CAD build for the part. Positions are in the model's coordinates, mm. A direction names the side the tool comes from. Give positions to 0.01 mm unless a question says otherwise; leave off trailing zeros. Loops run counter-clockwise (first coordinate to the right, second up) from the corner with the lowest first, then second, coordinate; pieces in that order, holes last.
Autodesk Inventor part; units mm, degrees
ref_plane "YZ Plane" through (0, 0, 0) normal (1, 0, 0) x (0, 1, 0)
ref_plane "XZ Plane" through (0, 0, 0) normal (0, 1, 0) x (-1, 0, 0)
ref_plane "XY Plane" through (0, 0, 0) normal (0, 0, 1) x (1, 0, 0)
sketch "Sketch1" plane through (0, 0, 0) normal (0, 0, 1) x (1, 0, 0)
  circle A0 centre (0, 0) radius 3.175
  dimension "d0" = 6.35
extrude "Extrusion1" add sketch "Sketch1" along normal blind 12.7
sketch "Sketch2" plane through (0, 0, 12.7) normal (0, 0, 1) x (1, 0, 0)
  circle A0 centre (0, 0) radius 6.35
  dimension "d3" = 12.7
extrude "Extrusion2" add sketch "Sketch2" along normal blind 25.4
sketch "Sketch3" plane through (0, 0, 38.1) normal (0, 0, 1) x (1, 0, 0)
  circle A0 centre (0, 0) radius 6.35
sketch "Sketch4" plane through (0, 0, 38.1) normal (0, 0, 1) x (1, 0, 0)
  point P0 (0, 0)
hole "Hole2" at (0, 0, 38.1) direction (0, 0, -1) diameter 4.9784 depth 22.225 tip angle 118
properties part number "Pin" material "Aluminum 6061"
1. Saw through at A-A, the plane z = 16.5. List the corners of the cut face in (x, y), and give its area (3 significant figures).
Responses:
outline: circle Ø12.7 at (0, 0); hole circle Ø4.98 at (0, 0)
area: 107 mm2
2. Saw through at B-B, the plane y = -4. List the corners of the cut face in (x, z).
Responses:
outline: (-4.93, 12.7) - (4.93, 12.7) - (4.93, 38.1) - (-4.93, 38.1) - close
3. Drop flat-ended pins along their axis: pin 1 (3 mm diameter, centred on y = 3.5, z = 27, fed in from +X); pin 2 (2 mm diameter, centred on y = 4, z = 15, fed in from +X); pin 3 (6 mm diameter, centred on x = 2.5, y = -1, fed in from -Z); pin 4 (1 mm diameter, centred on y = -1, z = 11.5, fed in from +X). Give the stop position or say it passes through.
Responses:
pin 1: stops at x = 6.03
pin 2: stops at x = 5.6
pin 3: stops at z = 0
pin 4: stops at x = 3.14
4. Saw through at C-C, the plane z = 10. List the corners of the cut face in (x, y) (3 decimals).
Responses:
outline: circle Ø6.35 at (0, 0)
5. Tool access for faces 4 (the face through (-0.69, 3.1, 6.26)), 5 (the face through (-0.422, 0.094, 14.639)): list every direction of +Z, -Z, +X, -X, +Y, -Y with a clear straight run to the whole face (end or side of a thin tool).
Responses:
face 4: -Z
face 5: +Z
6. Probe line 1 along Y through (x, z) = (0, 28); line 2 along Z through (x, y) = (-0.25, -3.75); line 3 along X through (y, z) = (-5.5, 28.5). List the from-to ranges inside material, lowest first.
Responses:
line 1: y = -6.35 to -2.49, 2.49 to 6.35
line 2: z = 12.7 to 38.1
line 3: x = -3.17 to 3.17
7. Pull direction X, two halves, no side cores. Call faces 1 (the face through (-1.38, 6.2, 25.22)), 2 (the face through (3, 0, 38.1)), 3 (the face through (-0.748, -2.374, 26.832)): released by +X, released by -X, zero draft, split by the parting line, or undercut.
Responses:
face 1: split by the parting line
face 2: zero draft
face 3: undercut
8. Saw through at D-D, the plane x = -3.75. List the corners of the cut face in (y, z), and give its area (3 significant figures).
Responses:
outline: (-5.12, 12.7) - (5.12, 12.7) - (5.12, 38.1) - (-5.12, 38.1) - close
area: 260 mm2
